Read the model definition and answer for the solid it produces. Units are mm, in the model's axes. A direction names the side the tool comes from. Coordinates: 2 decimals unless noted, no trailing zeros. Order: outer loops, then holes, each group sorted by start corner. A loop starts at its lowest first (then second) coordinate and runs counter-clockwise, first axis right, second up.
from build123d import *

# Parameters (mm, degrees)
SKETCH_W        = 22.7
SKETCH_H        = 12.2
PAD_DEPTH       = 18.3
PAD001_DEPTH    = 2.7
SKETCH002_W     = 22.7
SKETCH002_H     = 12.2
PAD002_DEPTH    = 4.5
PAD003_DEPTH    = 5.7
SKETCH004_R     = 2.5
POCKET_DEPTH    = 10
POCKET001_DEPTH = 1
SKETCH010_W     = 20.2
SKETCH010_H     = 10.2
POCKET003_DEPTH = 0.2


with BuildPart() as part:
    # Sketch → Pad (new body)
    with BuildSketch(Plane.XY):
        with Locations((-5.45, 0)):
            Rectangle(SKETCH_W, SKETCH_H)
    extrude(amount=-PAD_DEPTH)

    # Sketch001 → Pad001 (join)
    with BuildSketch(Plane.XY):
        with BuildLine():
            Line((-21.6, 6.1), (-21.6, 0.6))
            Line((-20.25, 0.6), (-21.6, 0.6))
            ThreePointArc((-20.25, -0.6), (-18.45, 0), (-20.25, 0.6))
            Line((-20.25, -0.6), (-21.6, -0.6))
            Line((-21.6, -0.6), (-21.6, -6.1))
            Line((-21.6, -6.1), (10.7, -6.1))
            Line((10.7, -6.1), (10.7, -0.6))
            Line((9.35, -0.6), (10.7, -0.6))
            ThreePointArc((9.35, 0.6), (7.55, 0), (9.35, -0.6))
            Line((9.35, 0.6), (10.7, 0.6))
            Line((10.7, 0.6), (10.7, 6.1))
            Line((10.7, 6.1), (-21.6, 6.1))
        make_face()
    extrude(amount=PAD001_DEPTH)

    # Sketch002 → Pad002 (join)
    with BuildSketch(Plane.XY):
        with Locations((-5.45, 0)):
            Rectangle(SKETCH002_W, SKETCH002_H)
    extrude(amount=PAD002_DEPTH)

    # Sketch003 (on Face18 of Pad002) → Pad003 (join)
    with BuildSketch(Plane.XY.offset(4.5)):
        with BuildLine():
            ThreePointArc((-5.307407, -2.798469), (6, 0), (-5.307407, 2.798469))
            ThreePointArc((-5.307407, 2.798469), (-8.2, 0), (-5.307407, -2.798469))
        make_face()
    extrude(amount=PAD003_DEPTH)

    # Sketch004 → Pocket (cut)
    with BuildSketch(Plane.XY.offset(5)):
        Circle(SKETCH004_R)
    extrude(amount=POCKET_DEPTH, mode=Mode.SUBTRACT)

    # Sketch005 (on Face10 of Pocket) → Pocket001 (cut)
    with BuildSketch(Plane.YZ.offset(5.9)):
        with BuildLine():
            ThreePointArc((-1.25, -12.65), (-1.9, -13.3), (-1.25, -13.95))
            Line((-1.25, -13.95), (1.25, -13.95))
            ThreePointArc((1.25, -13.95), (1.9, -13.3), (1.25, -12.65))
            Line((1.25, -12.65), (-1.25, -12.65))
        make_face()
    extrude(amount=-POCKET001_DEPTH, mode=Mode.SUBTRACT)

    # Sketch010 (on Face14 of Pocket001) → Pocket003 (cut)
    with BuildSketch(Plane.XZ.offset(6.1)):
        with Locations((-5.45, -8.2)):
            Rectangle(SKETCH010_W, SKETCH010_H)
    pocket003 = extrude(amount=-POCKET003_DEPTH, mode=Mode.SUBTRACT)

    # Mirrored: Pocket003 across XZ
    add(pocket003.mirror(Plane.XZ), mode=Mode.SUBTRACT)


solid = part.part
Q1. The part is cut by section B-B, the plane x = -13.5. Determine the outline of the cut face in (y, z).
Q2. Each of these flat-tipped pins is pushed along its axis until it touches: P1, Ø2, axis at y = -2.5, z = 4, coming from the -X side; P2, Ø3.5, axis at y = -1, z = -11.5, coming from the +X side; P3, Ø1.5, axis at y = 1, z = 7, coming from the -X side. Where does it stop, or does it pass through?
Q3. The part is cut by section D-D, the plane y = 0. Determine the outline of the cut face in (x, z), then the cut area to 3 significant figures.
Q4. The part is cut by section C-C, the plane x = 8.5. Determine the outline of the cut face in (y, z), then the cut area to 3 significant figures.
Q5. Which of the six approach directions +Z, -Z, +X, -X, +Y, -Y give full straight-line access (tool end or side, diameter ignored) to faces 1 (the flat face through (-18, 0, 0)), 2 (the flat face through (-16.8, 0, 4)), 3 (the flat face through (10, 0.6, 1))?
Q6. The part is cut by section A-A, the plane z = -8.5. Determine the outline of the cut face in (x, y), then the cut area to 3 significant figures.
Q7. Determine the mould class of faces 4 (the flat face through (-6, -5.9, -8)), 5 (the flat face through (0, 0, 5)), 6 (the cylindrical face through (-0.54, -2.44, 7.56)) for opening direction Z: +Z half, -Z half, draft (parallel to the pull), parting line (faces both ways), or undercut.
Q8. Straight lines are drawn through the part: L1, parallel to X at y = 0, z = 8.35; L2, parallel to Y at x = 0, z = 8; L3, parallel to Z at x = -5.5, y = -3.75. For each, find the intervals that lie inside material, in ascending order.
Computed values:
1. outline: (-6.1, -18.3) - (6.1, -18.3) - (6.1, -13.3) - (5.9, -13.3) - (5.9, -3.1) - (6.1, -3.1) - (6.1, 4.5) - (-6.1, 4.5) - (-6.1, -3.1) - (-5.9, -3.1) - (-5.9, -13.3) - (-6.1, -13.3) - close
2. P1: stops at x = -16.8
2. P2: stops at x = 5.9
2. P3: stops at x = -8.19
3. outline: (-18.45, 0) - (-16.8, 0) - (-16.8, -18.3) - (5.9, -18.3) - (5.9, -13.95) - (4.9, -13.95) - (4.9, -12.65) - (5.9, -12.65) - (5.9, 0) - (7.55, 0) - (7.55, 2.7) - (5.9, 2.7) - (5.9, 4.5) - (6, 4.5) - (6, 10.2) - (2.5, 10.2) - (2.5, 5) - (-2.5, 5) - (-2.5, 10.2) - (-8.2, 10.2) - (-8.2, 4.5) - (-16.8, 4.5) - (-16.8, 2.7) - (-18.45, 2.7) - close
3. area: 580 mm2
4. outline: (-6.1, 0) - (-1, 0) - (-1, 2.7) - (-6.1, 2.7) - close; (1, 0) - (6.1, 0) - (6.1, 2.7) - (1, 2.7) - close
4. area: 27.5 mm2
5. face 1: -Z, -X, +Y, -Y
5. face 2: +Z, -X, +Y, -Y
5. face 3: +Z, -Z, +X
6. outline: (-16.8, -6.1) - (-15.55, -6.1) - (-15.55, -5.9) - (4.65, -5.9) - (4.65, -6.1) - (5.9, -6.1) - (5.9, 6.1) - (4.65, 6.1) - (4.65, 5.9) - (-15.55, 5.9) - (-15.55, 6.1) - (-16.8, 6.1) - close
6. area: 269 mm2
7. face 4: undercut
7. face 5: +Z half
7. face 6: draft
8. L1: x = -8.2 to -2.5, 2.5 to 6
8. L2: y = -6 to -2.5, 2.5 to 6
8. L3: z = -18.3 to 4.5
